Read the model definition and answer for the solid it produces. Units are mm, in the model's axes. Face numbers are marked on the shaded views. A direction names the side the tool comes from. Coordinates: 2 decimals unless noted, no trailing zeros. Order: outer loops, then holes, each group sorted by start corner. A loop starts at its lowest first (then second) coordinate and runs counter-clockwise, first axis right, second up. Notation, with made-up numbers: (-37, 34) -> (13, 34) arc R8 ccw to (13, 41) -> close; hole circle Ø9 at (49, 43). An arc over 180 degrees is marked (long way). Return JSON: item names as keys, results as strings. Group by question number.
```python
from build123d import *

# Parameters (mm, degrees)
SKETCH_R        = 1.7
PAD_DEPTH       = 5
PAD001_DEPTH    = 10
SKETCH002_R     = 2.6
POCKET_DEPTH    = 15
POCKET001_DEPTH = 9
SKETCH004_R     = 1.8
POCKET002_DEPTH = 8
POCKET003_DEPTH = 2


with BuildPart() as part:
    # Sketch → Pad (new body)
    with BuildSketch(Plane.XY):
        with BuildLine():
            ThreePointArc((10, 20), (0, 10.000015), (9.99997, 0))
            Line((9.99997, 0), (39.99997, 0))
            ThreePointArc((39.99997, 0), (49.999939, 10.000015), (39.999939, 20))
            Line((10, 20), (39.999939, 20))
        make_face()
        with Locations((39.999939, 10)):
            Circle(SKETCH_R, mode=Mode.SUBTRACT)
        with Locations((10, 10)):
            Circle(SKETCH_R, mode=Mode.SUBTRACT)
    extrude(amount=PAD_DEPTH)

    # Sketch001 → Pad001 (new body)
    with BuildSketch(Plane.XY.offset(5)):
        with BuildLine():
            ThreePointArc((28, 0.460608), (34.633202, 7.316453), (32.5, 16.614378))
            Line((17.5, 16.614378), (32.5, 16.614378))
            ThreePointArc((17.5, 16.614378), (15.366798, 7.316453), (22, 0.460608))
            Line((22, 0.460608), (28, 0.460608))
        make_face()
    extrude(amount=PAD001_DEPTH)

    # Sketch002 → Pocket (cut)
    with BuildSketch(Plane.XY.offset(15)):
        with Locations((25, 10)):
            Circle(SKETCH002_R)
    extrude(amount=-POCKET_DEPTH, mode=Mode.SUBTRACT)

    # Sketch003 → Pocket001 (cut)
    with BuildSketch(Plane.XY.offset(15)):
        Polygon((22, 6), (28, 6), (28, 4), (25, 4), (22, 4), align=None)
    extrude(amount=-POCKET001_DEPTH, mode=Mode.SUBTRACT)

    # Sketch004 → Pocket002 (cut)
    with BuildSketch(Plane.XZ.offset(-0.460608)):
        with Locations((25, 11)):
            Circle(SKETCH004_R)
    extrude(amount=-POCKET002_DEPTH, mode=Mode.SUBTRACT)

    # Sketch005 → Pocket003 (cut)
    with BuildSketch(Plane.XY.offset(5)):
        Polygon((6.998384, 8.267949), (6.998384, 11.732051), (9.998384, 13.464102), (12.998384, 11.732051), (12.998384, 8.267949), (9.998384, 6.535898), align=None)
        Polygon((39.999999, 13.464101), (43, 11.732051), (43, 8.267949), (40, 6.535897), (37, 8.267948), (37, 11.73205), align=None)
    extrude(amount=-POCKET003_DEPTH, mode=Mode.SUBTRACT)


solid = part.part
```
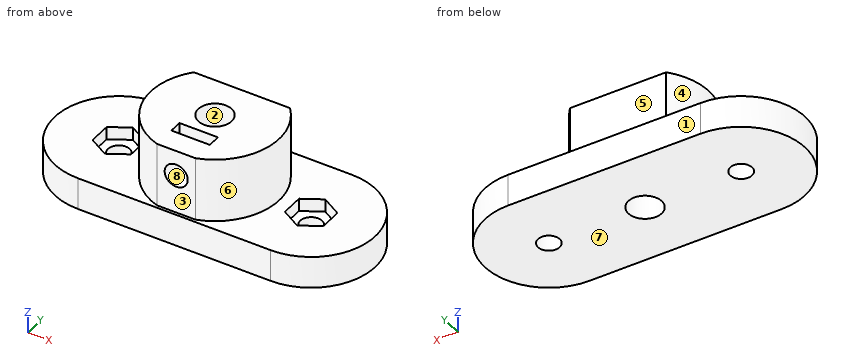
1. Which of the six approach directions +Z, -Z, +X, -X, +Y, -Y give full straight-line access (tool end or side, diameter ignored) to the marked faces 4, 5, 6, 7 and 8?
2. Find section D-D on x = 9. Determine the outline of the cut face in (y, z), and give its area (3 significant figures).
3. Find section C-C on x = 25. Determine the outline of the cut face in (y, z), and give its area (3 significant figures).
4. Straight lines are drawn through the part: L1, parallel to Z at x = 25, y = 1.85; L2, parallel to Y at x = 10, z = 1.9; L3, parallel to Z at x = 40.5, y = 2. For each, find the intervals that lie inside material, in ascending order.
5. For a pull along Y with two mould halves and no side action, classify the marked faces 1, 2 and 3 as released by +Y, released by -Y, zero draft, split by the parting line, or undercut.
6. Given pin 1 (4.5 mm diameter, centred on x = 25, z = 11, fed in from +Y); pin 2 (1 mm diameter, centred on x = 24.5, y = 5, fed in from +Z); pin 3 (1.8 mm diameter, centred on x = 41.5, y = 9.5, fed in from +Z), each flat-ended and moving along its own axis, determine where each tip first touches the part or whether it passes through.
7. Find section A-A on y = 10. Determine the outline of the cut face in (x, z).
8. Find section B-B on z = 2.5. Determine the outline of the cut face in (x, y).
Result:
{
 "1": {"face 4": "+Z, -X", "face 5": "+Z, +X, -X, +Y", "face 6": "+Z, +X", "face 7": "-Z, +X, -X, +Y, -Y", "face 8": "-Y"},
 "2": {"outline": "(0.05, 0) -> (8.63, 0) -> (8.63, 3) -> (7.11, 3) -> (7.11, 5) -> (0.05, 5) -> close; (11.37, 0) -> (19.95, 0) -> (19.95, 5) -> (12.89, 5) -> (12.89, 3) -> (11.37, 3) -> close", "area": "79.7 mm^2"},
 "3": {"outline": "(0, 0) -> (7.4, 0) -> (7.4, 9.2) -> (6, 9.2) -> (6, 6) -> (4, 6) -> (4, 9.2) -> (0.46, 9.2) -> (0.46, 5) -> (0, 5) -> close; (0.46, 12.8) -> (4, 12.8) -> (4, 15) -> (0.46, 15) -> close; (6, 12.8) -> (7.4, 12.8) -> (7.4, 15) -> (6, 15) -> close; (12.6, 0) -> (20, 0) -> (20, 5) -> (16.61, 5) -> (16.61, 15) -> (12.6, 15) -> close", "area": "148 mm^2"},
 "4": {"L1": "0 to 9.2, 12.8 to 15", "L2": "0 to 8.3, 11.7 to 20", "L3": "0 to 5"},
 "5": {"face 1": "released by +Y", "face 2": "undercut", "face 3": "released by -Y"},
 "6": {"pin 1": "y = 16.61", "pin 2": "z = 6", "pin 3": "z = 3"},
 "7": {"outline": "(0, 0) -> (8.3, 0) -> (8.3, 3) -> (7, 3) -> (7, 5) -> (0, 5) -> close; (11.7, 0) -> (22.4, 0) -> (22.4, 15) -> (15, 15) -> (15, 5) -> (13, 5) -> (13, 3) -> (11.7, 3) -> close; (27.6, 0) -> (38.3, 0) -> (38.3, 3) -> (37, 3) -> (37, 5) -> (35, 5) -> (35, 15) -> (27.6, 15) -> close; (41.7, 0) -> (50, 0) -> (50, 5) -> (43, 5) -> (43, 3) -> (41.7, 3) -> close"},
 "8": {"outline": "(10, 0) -> (40, 0) arc R10 ccw to (40, 20) -> (10, 20) arc R10 ccw to start; hole circle Ø3.4 at (10, 10); hole circle Ø5.2 at (25, 10); hole circle Ø3.4 at (40, 10)"}
}
